Part model, mm, in its own coordinate system. A direction names the side the tool comes from. Give positions to 0.01 mm unless a question says otherwise; leave off trailing zeros. Answer as CSV lines item,"result". Start each with the question number.
Item 1: Two-plate mould, pull along X, no slides. Class faces 4 (the flat face through (0, 250, 6)), 5 (the cylindrical face through (50.62, 227.27, 15.3)), 6 (the flat face through (-50.9, -205.6, 6)): +X half, -X half, draft (parallel to the pull), parting line (faces both ways), or undercut.
Item 2: Wall check: L1, parallel to Z at x = -5.5, y = 18.5; L2, parallel to Z at x = -34, y = 13.5; L3, parallel to X at y = 101.5, z = 19. Give the ranges that are in metal, low to high. Write a range as from..to.
Item 3: Band-saw the part on A-A, the plane y = -181. Count the separate pieces of the cut face and the enclosed holes in it, then the cut area to 3 significant figures.
Item 4: Pin check, flat tips, straight feed: pin 1 (10 mm diameter, centred on x = 32.5, y = -23.5, fed in from +Z); pin 2 (5 mm diameter, centred on x = -32, y = 43, fed in from -Z); pin 3 (1.9 mm diameter, centred on y = -146.5, z = 5, fed in from -X). Stop position of each tip, or through.
Item 5: 3-axis set-ups, long thin cutter, end or side, ignore diameter. For faces 1 (the flat face through (50.96, -205.52, 15.07)), 2 (the flat face through (0, 235, 32.864)), 3 (the flat face through (0, 65, 19.564)): which of +Z, -Z, +X, -X, +Y, -Y reach the whole face in a straight line?
from build123d import *

# Parameters (mm, degrees)
F1_DEPTH       = 250
F2_W           = 38
F2_H           = 13
F3_DEPTH       = 250
F4_T1_DEPTH    = 509.3674969976
F5_R           = 9
F7_DEPTH       = 500.001
F9_DEPTH       = 0.9604886552
F9_DEPTH_BACK  = 22.8653446865
F11_DEPTH      = 0.9604887634
F11_DEPTH_BACK = 22.8653447865
F13_DEPTH      = 15
F14_R          = 27.5
F15_DEPTH      = 100
F17_D          = 40
F19_D          = 8
F19_DEPTH      = 78.501
F21_DEPTH      = 72.501


# Not quite as in the source:
# - a fillet or chamfer that OpenCascade refuses, or shapes differently, is made with other operations: its cross-section is extruded or revolved along the edge and cut away or added


with BuildPart() as f1:
    # F0 (on Front) → F1 (new body, symmetric)
    with BuildSketch(Plane.XZ):
        with BuildLine():
            Line((22.5, 21.5643446865), (0, 21.5643446865))
            Line((0, 21.5643446865), (-22.5, 21.5643446865))
            Line((-22.5, 21.5643446865), (-22.5, 22.8643446865))
            Line((-22.5, 22.8643446865), (-43.8217498065, 22.8643446865))
            Line((-43.8217498065, 22.8643446865), (-57.5, 12.151993139))
            Line((-57.5, 12.151993139), (-57.5, 8.151993139))
            Line((-57.5, 8.151993139), (-37.5, -1.1356553135))
            ThreePointArc((-37.5, -1.1356553135), (0, 0.564188832), (37.5, -1.1356553135))
            Line((37.5, -1.1356553135), (57.5, 8.151993139))
            Line((57.5, 8.151993139), (57.5, 12.151993139))
            Line((57.5, 12.151993139), (43.8217498065, 22.8643446865))
            Line((43.8217498065, 22.8643446865), (22.5, 22.8643446865))
            Line((22.5, 22.8643446865), (22.5, 21.5643446865))
        make_face()
    extrude(amount=F1_DEPTH, both=True)

    # F2 (on Front) → F3 (cut, symmetric)
    with BuildSketch(Plane.XZ):
        with Locations((0, 13.0643446865)):
            Rectangle(F2_W, F2_H)
    extrude(amount=F3_DEPTH, both=True, mode=Mode.SUBTRACT)

    # F4: fillet of radius 2 on 2 edges, made by hand

    # F4_s2 → F4_t1 (cut)
    with BuildSketch(Plane.XZ.offset(-254.6837484988)):
        with BuildLine():
            ThreePointArc((-24.3734993995, 22.8643446865), (-23.2333239744, 22.507512359), (-22.5, 21.5643446865))
            Line((-22.5, 21.5643446865), (-22.5, 22.8643446865))
            Line((-22.5, 22.8643446865), (-24.3734993995, 22.8643446865))
        make_face()
        with BuildLine():
            ThreePointArc((24.3734993995, 22.8643446865), (23.2333239744, 22.507512359), (22.5, 21.5643446865))
            Line((22.5, 21.5643446865), (22.5, 22.8643446865))
            Line((22.5, 22.8643446865), (24.3734993995, 22.8643446865))
        make_face()
    extrude(amount=F4_T1_DEPTH, mode=Mode.SUBTRACT)

    # F5
    f5_edges = [f1.edges().sort_by_distance(p)[0] for p in [
        (43.82175, 0, 22.864345),
        (-43.82175, 0, 22.864345),
        (-37.5, 0, -1.135655),
        (37.5, 0, -1.135655),
    ]]
    fillet(f5_edges, radius=F5_R)

    # F6 (on face) → F7 (cut, through all)
    with BuildSketch(Plane.XZ.offset(250)):
        with BuildLine():
            ThreePointArc((-38.8398592766, 1.6916831032), (-37.1099744385, 1.1473623621), (-35.2983129545, 1.0656966447))
            ThreePointArc((-35.2983129545, 1.0656966447), (-28.1533234397, 1.6115661831), (-21, 2.034428437))
            Line((-21, 2.034428437), (-21, 19.5643446865))
            Line((-21, 19.5643446865), (-23, 19.5643446865))
            ThreePointArc((-23, 19.5643446865), (-23.7333239744, 20.507512359), (-24.8734993995, 20.8643446865))
            Line((-24.8734993995, 20.8643446865), (-40.7169256034, 20.8643446865))
            ThreePointArc((-40.7169256034, 20.8643446865), (-42.9997645145, 20.4816437205), (-45.0329906666, 19.3753865454))
            Line((-45.0329906666, 19.3753865454), (-55.617097211, 11.0862656041))
            ThreePointArc((-55.617097211, 11.0862656041), (-55.9939317717, 10.1844048326), (-55.4216999505, 9.3919984469))
            Line((-55.4216999505, 9.3919984469), (-38.8398592766, 1.6916831032))
        make_face()
        with BuildLine():
            Line((21, 19.5643446865), (21, 2.034428437))
            ThreePointArc((21, 2.034428437), (28.1533234397, 1.6115661831), (35.2983129545, 1.0656966447))
            ThreePointArc((35.2983129545, 1.0656966447), (37.1099744385, 1.1473623621), (38.8398592766, 1.6916831032))
            Line((38.8398592766, 1.6916831032), (55.4216999505, 9.3919984469))
            ThreePointArc((55.4216999505, 9.3919984469), (55.9939317717, 10.1844048326), (55.617097211, 11.0862656041))
            Line((55.617097211, 11.0862656041), (45.0329906666, 19.3753865454))
            ThreePointArc((45.0329906666, 19.3753865454), (42.9997645145, 20.4816437205), (40.7169256034, 20.8643446865))
            Line((40.7169256034, 20.8643446865), (24.8734993995, 20.8643446865))
            ThreePointArc((24.8734993995, 20.8643446865), (23.7333239744, 20.507512359), (23, 19.5643446865))
            Line((23, 19.5643446865), (21, 19.5643446865))
        make_face()
    extrude(amount=-F7_DEPTH, mode=Mode.SUBTRACT)

    # F8 (on Top) → F9 (cut, two sides)
    with BuildSketch(Plane.XY) as f9_sk:
        with BuildLine():
            ThreePointArc((-57.4987473195, 200.3795480055), (0, 257.5), (57.4987473195, 200.3795480055))
            Line((57.4987473195, 200.3795480055), (56.9706690247, 280.3795480055))
            Line((56.9706690247, 280.3795480055), (-56.9706690247, 280.3795480055))
            Line((-56.9706690247, 280.3795480055), (-57.4987473195, 200.3795480055))
        make_face()
    extrude(amount=-F9_DEPTH, mode=Mode.SUBTRACT)
    extrude(f9_sk.sketch, amount=F9_DEPTH_BACK, mode=Mode.SUBTRACT)

    # F10 (on Top) → F11 (cut, two sides)
    with BuildSketch(Plane.XY) as f11_sk:
        Polygon((-16, -216.0670316956), (-43.2975540478, -216.0670316956), (-68, -182.0670316956), (-68, -312.0670316956), (0, -312.0670316956), (0, -106.0670316956), (-16, -106.0670316956), align=None)
        Polygon((16, -106.0670316956), (0, -106.0670316956), (0, -312.0670316956), (68, -312.0670316956), (68, -182.0670316956), (43.2975540478, -216.0670316956), (16, -216.0670316956), align=None)
    extrude(amount=-F11_DEPTH, mode=Mode.SUBTRACT)
    extrude(f11_sk.sketch, amount=F11_DEPTH_BACK, mode=Mode.SUBTRACT)

    # F12 (on Right) → F13 (join, symmetric)
    with BuildSketch(Plane.YZ):
        with BuildLine():
            ThreePointArc((297.0295354887, 181.5643446865), (245.7826981398, 96.2483289481), (180, 21.5643446865))
            Line((180, 21.5643446865), (250, 21.5643446865))
            ThreePointArc((250, 21.5643446865), (267.5395947829, 67.9098502341), (311.3687395561, 91.0301732869))
            Line((311.3687395561, 91.0301732869), (312.6729819927, 82.795510627))
            Line((312.6729819927, 82.795510627), (358.1066456601, 89.9914960188))
            Line((358.1066456601, 89.9914960188), (342.4631991561, 188.7603300783))
            Line((342.4631991561, 188.7603300783), (297.0295354887, 181.5643446865))
        make_face()
    extrude(amount=F13_DEPTH, both=True)

    # F14 (on face) → F15 (join, through all)
    with BuildSketch(Plane(origin=(0, -20.7844039253, 131.2275617651), x_dir=(1, 0, 0), z_dir=(0, -0.156434465, 0.9876883406))):
        with Locations((0, 344.775530146)):
            Circle(F14_R)
    extrude(amount=-F15_DEPTH)

    # F17 (through all)
    with Locations(Plane(origin=(0, -20.7844039253, 131.2275617651), x_dir=(1, 0, 0), z_dir=(0, -0.156434465, 0.9876883406))):
        with Locations((0, 344.775530146)):
            Hole(F17_D / 2)

    # F19 (through all, one way)
    with BuildSketch(Plane.YZ.offset(21)):
        with Locations((-202.0670316956, 12.034428437)):
            Circle(F19_D / 2)
    extrude(amount=-F19_DEPTH, mode=Mode.SUBTRACT)

    # F20 (on face) → F21 (cut, through all)
    with BuildSketch(Plane.YZ.offset(15)):
        with BuildLine():
            Line((303.3300998051, 106.5364009657), (296.8697635571, 130.2439192545))
            ThreePointArc((296.8697635571, 130.2439192545), (292.1354764945, 133.9285390129), (287.271901756, 130.4163406247))
            Line((287.271901756, 130.4163406247), (278.5350250255, 102.3679551307))
            ThreePointArc((278.5350250255, 102.3679551307), (279.7315404872, 97.3876414374), (284.6820479704, 96.0732406641))
            Line((284.6820479704, 96.0732406641), (299.8792609489, 100.4141078692))
            ThreePointArc((299.8792609489, 100.4141078692), (302.8617375272, 102.7667124398), (303.3300998051, 106.5364009657))
        make_face()
        with BuildLine():
            ThreePointArc((243.4909897109, 32.8643446865), (246.3588718926, 33.768584465), (248.1894528148, 36.1542439699))
            Line((248.1894528148, 36.1542439699), (255.8716915251, 57.2610213573))
            ThreePointArc((255.8716915251, 57.2610213573), (254.0207530146, 63.0810616952), (247.921439605, 62.7692623419))
            Line((247.921439605, 62.7692623419), (223.2683930345, 41.6624849544))
            ThreePointArc((223.2683930345, 41.6624849544), (221.8302617373, 36.1309522525), (226.5201818507, 32.8643446865))
            Line((226.5201818507, 32.8643446865), (243.4909897109, 32.8643446865))
        make_face()
    extrude(amount=-F21_DEPTH, mode=Mode.SUBTRACT)


solid = f1.part
Output:
1,face 4,"draft"
1,face 5,"undercut"
1,face 6,"-X half"
2,L1,"0.53..6.56, 19.56..21.56"
2,L2,"-0.83..1.17, 20.86..22.86"
2,L3,"-48.76..-45.51, -21..-19, 19..21, 45.51..48.76"
3,separate pieces,"2"
3,enclosed holes,"2"
3,area,"453 mm²"
4,pin 1,"z = 22.86"
4,pin 2,"z = -0.87"
4,pin 3,"x = -52.76"
5,face 1,"+Z, -Z, +X, -Y"
5,face 2,"+X, -X"
5,face 3,"+Y, -Y"
